For this review, take the finished solid that the model builds, in its own axes (mm). A direction names the side the tool comes from. Give positions to 0.01 mm unless a question says otherwise; leave off trailing zeros. Loops run counter-clockwise (first coordinate to the right, second up) from the corner with the lowest first, then second, coordinate; pieces in that order, holes last. Notation, with made-up numbers: (34.25, 16) -> (60.25, 16) arc R34 ccw to (60.25, 46) -> close; hole circle Ø3 at (2.5, 52). An arc over 180 degrees is marked (long way). Answer as CSV lines item,"result". Start each with the question number.
Item 1: Add section C-C on y = 20. State how many separate pieces and enclosed holes the cut face has, plus the area to 3 significant figures.
Item 2: Add section B-B on x = 9.25. State the section outline as (y, z) points.
Item 3: For L1, parallel to X at y = 23.25, z = 225.5; L2, parallel to Y at x = 29.25, z = 15, list the stretches that pass through material, from the lowest coordinate up. Write a range as from..to.
Item 4: The part is to be moulded in two halves that separate along X. For faces 3 (the face through (0, 1, 123)), 4 (the face through (15, 30, 123)), 5 (the face through (1.5, 3, 123)), say which applies: +X half, -X half, draft (parallel to the pull), parting line (faces both ways), or undercut.
Item 5: Clearance check with flat-ended pins moving along their axes: P1, Ø4, axis at x = 21, z = 95.5, coming from the -Y side; P2, Ø4.5, axis at y = 15, z = 235, coming from the +X side. State where each tip first meets the part, or that it passes through.
Item 6: Machinability: for faces 1 (the face through (14, 1, 0)), 2 (the face through (28.5, 3, 123)), which of the approach directions +Z, -Z, +X, -X, +Y, -Y give a long, thin tool a straight path to every point of the face, cutting with its end or side? Answer none if there is none.
Item 7: Add section D-D on z = 235. State the section outline as (x, y) points, plus the area to 3 significant figures.
Item 8: Add section A-A on z = 75. State the section outline as (x, y) points, plus the area to 3 significant figures.
```python
from build123d import *

# Parameters (mm, degrees)
SKETCH1_W           = 30
SKETCH1_H           = 30
SKETCH1_W_2         = 27
SKETCH1_H_2         = 27
BOSS_EXTRUDE1_DEPTH = 250
SKETCH2_R           = 3.1
SKETCH2_R_2         = 2.5
SKETCH2_R_3         = 11.5
SKETCH2_R_4         = 1.75
CUT_EXTRUDE1_DEPTH  = 254.574446662
SKETCH3_R           = 2.2
CUT_EXTRUDE2_DEPTH  = 254.574446662


with BuildPart() as part:
    # Sketch1 → Boss-Extrude1 (new body)
    with BuildSketch(Plane.XY):
        with Locations((15, 15)):
            Rectangle(SKETCH1_W, SKETCH1_H)
        with Locations((15, 15)):
            Rectangle(SKETCH1_W_2, SKETCH1_H_2, mode=Mode.SUBTRACT)
    extrude(amount=BOSS_EXTRUDE1_DEPTH)

    # Sketch2 → Cut-Extrude1 (cut, through all)
    with BuildSketch(Plane(origin=(30, 0, 0), x_dir=(0, 0, -1), z_dir=(1, 0, 0))):
        with Locations((-75, 20)):
            Circle(SKETCH2_R)
        with Locations((-15, 15)):
            Circle(SKETCH2_R_2)
        with Locations((-235, 15)):
            Circle(SKETCH2_R_2)
        with Locations((-125, 15)):
            Circle(SKETCH2_R_3)
        with Locations((-146.92, 15)):
            Circle(SKETCH2_R_4)
        with Locations((-103.08, 15)):
            Circle(SKETCH2_R_4)
        with BuildLine():
            Line((-185, 23.1), (-165, 23.1))
            ThreePointArc((-165, 23.1), (-161.9, 20), (-165, 16.9))
            Line((-165, 16.9), (-185, 16.9))
            ThreePointArc((-185, 16.9), (-188.1, 20), (-185, 23.1))
        make_face()
    extrude(amount=-CUT_EXTRUDE1_DEPTH, mode=Mode.SUBTRACT)

    # Sketch3 → Cut-Extrude2 (cut, through all)
    with BuildSketch(Plane(origin=(0, 30, 0), x_dir=(1, 0, 0), z_dir=(0, 1, 0))):
        with Locations(Location((15, -25, 0), (0, 0, 270))):
            Circle(SKETCH3_R)
        with Locations(Location((15, -225, 0), (0, 0, 270))):
            Circle(SKETCH3_R)
    extrude(amount=-CUT_EXTRUDE2_DEPTH, mode=Mode.SUBTRACT)


solid = part.part
```
Computed values:
1,separate pieces,"8"
1,enclosed holes,"0"
1,area,"591 mm²"
2,outline,"(0, 0) -> (1.5, 0) -> (1.5, 250) -> (0, 250) -> close; (28.5, 0) -> (30, 0) -> (30, 250) -> (28.5, 250) -> close"
3,L1,"0..1.5, 28.5..30"
3,L2,"0..12.5, 17.5..30"
4,face 3,"-X half"
4,face 4,"draft"
4,face 5,"undercut"
5,P1,"y = 0"
5,P2,"through"
6,face 1,"-Z, +X, -X, +Y, -Y"
6,face 2,"+Z, -Z"
7,outline,"(0, 0) -> (30, 0) -> (30, 12.5) -> (28.5, 12.5) -> (28.5, 1.5) -> (1.5, 1.5) -> (1.5, 12.5) -> (0, 12.5) -> close; (0, 17.5) -> (1.5, 17.5) -> (1.5, 28.5) -> (28.5, 28.5) -> (28.5, 17.5) -> (30, 17.5) -> (30, 30) -> (0, 30) -> close"
7,area,"156 mm²"
8,outline,"(0, 0) -> (30, 0) -> (30, 16.9) -> (28.5, 16.9) -> (28.5, 1.5) -> (1.5, 1.5) -> (1.5, 16.9) -> (0, 16.9) -> close; (0, 23.1) -> (1.5, 23.1) -> (1.5, 28.5) -> (28.5, 28.5) -> (28.5, 23.1) -> (30, 23.1) -> (30, 30) -> (0, 30) -> close"
8,area,"152 mm²"
